```python
from build123d import *

# Parameters (mm, degrees)
ESQUISSE1_W             = 7.62
ESQUISSE1_H             = 2.54
BOSS_EXTRU_1_DEPTH      = 3
ESQUISSE2_R             = 0.3
ENL_V_MAT_EXTRU_1_DEPTH = 2
ESQUISSE3_R             = 0.7
BOSS_EXTRU_2_DEPTH      = 1
ESQUISSE4_R             = 0.3
BOSS_EXTRU_3_DEPTH      = 3
CHANFREIN1_SIZE         = 0.4


with BuildPart() as part:
    # Esquisse1 → Boss.-Extru.1 (new body)
    with BuildSketch(Plane(origin=(0, 0, 0), x_dir=(1, 0, 0), z_dir=(0, 1, 0))):
        Rectangle(ESQUISSE1_W, ESQUISSE1_H)
    extrude(amount=BOSS_EXTRU_1_DEPTH)

    # Esquisse2 → Enlèv. mat.-Extru.1 (cut)
    with BuildSketch(Plane(origin=(0, 3, 0), x_dir=(1, 0, 0), z_dir=(0, 1, 0))):
        with Locations(Location((-2.54, 0, 0), (0, 0, 270))):
            Circle(ESQUISSE2_R)
        with Locations(Location((0, 0, 0), (0, 0, 270))):
            Circle(ESQUISSE2_R)
        with Locations(Location((2.54, 0, 0), (0, 0, 270))):
            Circle(ESQUISSE2_R)
    extrude(amount=-ENL_V_MAT_EXTRU_1_DEPTH, mode=Mode.SUBTRACT)

    # Esquisse3 → Boss.-Extru.2 (add)
    with BuildSketch(Plane(origin=(0, 0, 0), x_dir=(1, 0, 0), z_dir=(0, 1, 0))):
        with Locations(Location((-2.54, 0, 0), (0, 0, 270))):
            Circle(ESQUISSE3_R)
        with Locations(Location((0, 0, 0), (0, 0, 270))):
            Circle(ESQUISSE3_R)
        with Locations(Location((2.54, 0, 0), (0, 0, 270))):
            Circle(ESQUISSE3_R)
    extrude(amount=-BOSS_EXTRU_2_DEPTH)

    # Esquisse4 → Boss.-Extru.3 (add)
    with BuildSketch(Plane.XZ.offset(1)):
        with Locations(Location((-2.54, 0, 0), (0, 0, 90))):
            Circle(ESQUISSE4_R)
        with Locations(Location((0, 0, 0), (0, 0, 90))):
            Circle(ESQUISSE4_R)
        with Locations(Location((2.54, 0, 0), (0, 0, 90))):
            Circle(ESQUISSE4_R)
    extrude(amount=BOSS_EXTRU_3_DEPTH)

    # Chanfrein1
    chanfrein1_edges = [part.edges().sort_by_distance(p)[0] for p in [
        (-2.54, 3, -0.3),
        (2.54, 3, -0.3),
        (0, 3, -0.3),
        (-2.54, -1, -0.3),
        (0, -1, -0.3),
        (2.54, -1, -0.3),
        (-3.81, 1.5, -1.27),
        (3.81, 1.5, -1.27),
        (3.81, 1.5, 1.27),
        (-3.81, 1.5, 1.27),
    ]]
    chamfer(chanfrein1_edges, length=CHANFREIN1_SIZE - 0.0001)  # a hair under: the kernel refuses the full size


solid = part.part
```
The model under review builds one solid part; all positions refer to its coordinate system, in mm. A direction names the side the tool comes from. Round coordinates to 2 decimals unless told otherwise and drop trailing zeros. Order: outer loops, then holes, each group sorted by start corner. A loop starts at its lowest first (then second) coordinate and runs counter-clockwise, first axis right, second up. Notation, with made-up numbers: (14, 2) - (57, 2) arc R19 cw to (57, 20) - close; hole circle Ø2 at (18.25, -5). An arc over 180 degrees is marked (long way). Answer in a Markdown table with one row per item.
(1) For line 1 (X direction, y = 1.85, z = 0); line 2 (X direction, y = -3, z = 0); line 3 (Y direction, x = 3.25, z = 0.75), list the stretches that pass through material, from the lowest coordinate up. Write a range as from..to.
Result set:
| item | result |
|---|---|
| line 1 | x = -3.81..-2.84, -2.24..-0.3, 0.3..2.24, 2.84..3.81 |
| line 2 | x = -2.84..-2.24, -0.3..0.3, 2.24..2.84 |
| line 3 | y = 0..3 |
(2) Mouldability with a two-part tool opening along X and no side actions: class faces 1 (the face through (0, -0.5, -0.7)), 2 (the face through (0, 1, -1.27)), 3 (the face through (3.81, 1, 0)), 4 (the face through (-1.846, -0.493, -0.091)) as released by +X, released by -X, zero draft, split by the parting line, or undercut.
Result set:
| item | result |
|---|---|
| face 1 | undercut |
| face 2 | zero draft |
| face 3 | released by +X |
| face 4 | undercut |
(3) Take a section at D-D on y = -0.75. Write out the cut boundary in (x, z).
Result set:
| item | result |
|---|---|
| outline | circle Ø1.4 at (-2.54, 0); circle Ø1.4 at (0, 0); circle Ø1.4 at (2.54, 0) |
(4) Take a section at B-B on y = -1.5. Write out the cut boundary in (x, z).
Result set:
| item | result |
|---|---|
| outline | circle Ø0.6 at (-2.54, 0); circle Ø0.6 at (0, 0); circle Ø0.6 at (2.54, 0) |
(5) Clearance check with flat-ended pins moving along their axes: P1, Ø0.7, axis at x = -2.5, z = 0, coming from the +Y side; P2, Ø0.5, axis at x = 0, z = 0, coming from the +Y side; P3, Ø1.5, axis at x = -2, y = -2.5, coming from the -Z side. State where each tip first meets the part, or that it passes through.
Result set:
| item | result |
|---|---|
| P1 | stops at y = 2.69 |
| P2 | stops at y = 1 |
| P3 | stops at z = -0.3 |
(6) Machinability: for faces 5 (the face through (-3.81, 1, 0)), 6 (the face through (1.857, -0.493, -0.152)), which of the approach directions +Z, -Z, +X, -X, +Y, -Y give a long, thin tool a straight path to every point of the face, cutting with its end or side? Answer none if there is none.
Result set:
| item | result |
|---|---|
| face 5 | +Z, -Z, -X, +Y, -Y |
| face 6 | -Y |
(7) Take a section at A-A on y = 2. Write out the cut boundary in (x, z).
Result set:
| item | result |
|---|---|
| outline | (-3.81, -0.87) - (-3.41, -1.27) - (3.41, -1.27) - (3.81, -0.87) - (3.81, 0.87) - (3.41, 1.27) - (-3.41, 1.27) - (-3.81, 0.87) - close; hole circle Ø0.6 at (-2.54, 0); hole circle Ø0.6 at (0, 0); hole circle Ø0.6 at (2.54, 0) |
